Check sheet for the modelled part. Datum: model origin and axes. Units: mm. A direction names the side the tool comes from. Give positions to 0.01 mm unless a question says otherwise; leave off trailing zeros. Order: outer loops, then holes, each group sorted by start corner. A loop starts at its lowest first (then second) coordinate and runs counter-clockwise, first axis right, second up.
```python
from build123d import *

# Parameters (mm, degrees)
SKETCH1_W               = 190
SKETCH1_H               = 50
BOSS_EXTRUDE1_DEPTH     = 120
SHELL1_T                = 5
SKETCH3_R               = 6.75
CUT_EXTRUDE2_DEPTH      = 242.091269025
CUT_EXTRUDE2_DEPTH_BACK = 242.091269025
M3_CLEARANCE_HOLE1_D    = 3.4
SKETCH8_R               = 7.5
CUT_EXTRUDE4_DEPTH      = 168.705098312
CUT_EXTRUDE4_DEPTH_BACK = 168.705098312
SKETCH10_W              = 13.4
SKETCH10_H              = 7.3
CUT_EXTRUDE6_DEPTH      = 5
FILLET1_R               = 3
SKETCH11_W              = 98.43460289
SKETCH11_H              = 30
REVOLVE1_ANGLE          = 15
CUT_EXTRUDE7_REACH      = 271.031
SKETCH12_R              = 2.2
M3_CLEARANCE_HOLE3_D    = 3.4


with BuildPart() as part:
    # Sketch1 → Boss-Extrude1 (new, symmetric)
    with BuildSketch(Plane.XY):
        with Locations((0, 25)):
            Rectangle(SKETCH1_W, SKETCH1_H)
    extrude(amount=BOSS_EXTRUDE1_DEPTH, both=True)

    # Shell1
    shell1_openings = [part.faces().sort_by_distance(p)[0] for p in [
        (0, 50, 0),
    ]]
    offset(amount=SHELL1_T, openings=shell1_openings, kind=Kind.INTERSECTION)

    # Sketch3 → Cut-Extrude2 (cut, two sides)
    with BuildSketch(Plane(origin=(100, 0, 0), x_dir=(0, 0, -1), z_dir=(1, 0, 0))) as cut_extrude2_sk:
        with Locations(Location((0, 20, 0), (0, 0, 270))):
            Circle(SKETCH3_R)
    extrude(amount=CUT_EXTRUDE2_DEPTH, mode=Mode.SUBTRACT)
    extrude(cut_extrude2_sk.sketch, amount=-CUT_EXTRUDE2_DEPTH_BACK, mode=Mode.SUBTRACT)

    # M3 Clearance Hole1 (through all)
    with Locations(Plane.XY.offset(125)):
        with Locations((-80.25, 42), (79.75, 42)):
            Hole(M3_CLEARANCE_HOLE1_D / 2)

    # Sketch8 → Cut-Extrude4 (cut, two sides)
    with BuildSketch(Plane(origin=(0, 0, 0), x_dir=(0, 0, -1), z_dir=(1, 0, 0))) as cut_extrude4_sk:
        with Locations((30, 25)):
            Circle(SKETCH8_R)
    extrude(amount=CUT_EXTRUDE4_DEPTH, mode=Mode.SUBTRACT)
    extrude(cut_extrude4_sk.sketch, amount=-CUT_EXTRUDE4_DEPTH_BACK, mode=Mode.SUBTRACT)

    # Sketch10 → Cut-Extrude6 (cut)
    with BuildSketch(Plane(origin=(0, 0, -125), x_dir=(-1, 0, 0), z_dir=(0, 0, -1))):
        with Locations((-15.8, 3.65)):
            Rectangle(SKETCH10_W, SKETCH10_H)
    extrude(amount=-CUT_EXTRUDE6_DEPTH, mode=Mode.SUBTRACT)

    # Fillet1
    fillet1_edges = [part.edges().sort_by_distance(p)[0] for p in [
        (22.5, 0, -122.5),
        (22.5, 7.3, -122.5),
        (9.1, 7.3, -122.5),
        (9.1, 0, -122.5),
    ]]
    fillet(fillet1_edges, radius=FILLET1_R)

    # Sketch11 → Revolve1 (revolve)
    with BuildSketch(Plane(origin=(0, 0, -125), x_dir=(-1, 0, 0), z_dir=(0, 0, -1))):
        with Locations((0, 35)):
            Rectangle(SKETCH11_W, SKETCH11_H)
    revolve(axis=Axis((49.217301445, 20, -125), (-1, 0, 0)), revolution_arc=REVOLVE1_ANGLE)

    # Cut-Extrude7: up to this plane
    cut_extrude7_end = Plane(origin=(0, 0, -120), z_dir=(0, 0, -1))
    # Sketch12 → Cut-Extrude7 (cut, up to the surface)
    with BuildSketch(Plane(origin=(0, -29.910254038, -111.626587737), x_dir=(-1, 0, 0), z_dir=(0, -0.25881904510252135, -0.9659258262890682)), mode=Mode.PRIVATE) as cut_extrude7_sk1:
        with Locations(Location((-37.5, 71.670897164, 0), (0, 0, 90))):
            Circle(SKETCH12_R)
    cut_extrude7_tool1 = split(extrude(cut_extrude7_sk1.sketch, amount=-CUT_EXTRUDE7_REACH, mode=Mode.PRIVATE), bisect_by=cut_extrude7_end, keep=Keep.BOTH, mode=Mode.PRIVATE)
    cut_extrude7 = cut_extrude7_tool1.solids().sort_by_distance((37.5, 39.318517, -130.176381))[0]
    add(cut_extrude7, mode=Mode.SUBTRACT)

    # Mirror2: Cut-Extrude7 across plane
    add(cut_extrude7.mirror(Plane(origin=(0, 0, 0), x_dir=(0, 0, 1), z_dir=(1, 0, 0))), mode=Mode.SUBTRACT)

    # M3 Clearance Hole3 (through all)
    with Locations(Plane(origin=(0, 5, 0), x_dir=(1, 0, 0), z_dir=(0, 1, 0))):
        with Locations((-47.903181707, 25), (-86.25, 25), (-47.903181707, -25), (-86.25, -25), (25, -49.28), (47.903181707, -25), (86.25, -25), (86.25, 25), (47.903181707, 25), (25, 31.75), (-25, 31.75), (-25, -49.28)):
            Hole(M3_CLEARANCE_HOLE3_D / 2)


solid = part.part
```
Q1. Go/stop test with flat-tipped pins: P1, Ø2, axis at x = -25, z = -31.75, coming from the -Y side; P2, Ø3, axis at x = 30, y = 10.5, coming from the -Z side; P3, Ø4, axis at x = -47.9, z = 25, coming from the +Y side; P4, Ø4, axis at y = 34.5, z = -129, coming from the +X side. Record where each tip stops, or that it passes through.
Q2. Sectioned sample at A-A, the plane z = 32.5. Record the cut outline in (x, y), plus the area to 3 significant figures.
Q3. Tool access check on faces 1 (the flat face through (-1, 17, -125)), 2 (the flat face through (16, 7.3, -123)), 3 (the flat face through (-1, 25, 120)), 4 (the flat face through (-49.217, 39, -128)). Record the directions out of +Z, -Z, +X, -X, +Y, -Y that give a thin tool (end or side, any length) a straight path to the whole face; none if there is none.
Q4. Draft check along X on faces 5 (the flat face through (49.217, 39, -128)), 6 (the flat face through (-1, -5, 2)), 7 (the flat face through (-1, 0, -1)). Enter one of: pulls with the +X half, pulls with the -X half, needs draft (parallel to the pull), parting line crosses it, or undercut.
Q5. Sectioned sample at B-B, the plane x = 5.5. Record the cut outline in (y, z), plus the area to 3 significant figures.
Q6. Material ranges on line 1 (X direction, y = -2.75, z = -25); line 2 (Z direction, x = 25, y = -1.9); line 3 (Z direction, x = 86.25, y = -2.35), recorded low to high.
Filled in:
1. P1: passes through
1. P2: stops at z = -125
1. P3: stops at y = 0
1. P4: stops at x = 49.22
2. outline: (-100, -5) - (100, -5) - (100, 50) - (95, 50) - (95, 0) - (-95, 0) - (-95, 50) - (-100, 50) - close
2. area: 1,500 mm2
3. face 1: -Z, -Y
3. face 2: -Z
3. face 3: +Y
3. face 4: -Z, -X, +Y, -Y
4. face 5: pulls with the +X half
4. face 6: needs draft
4. face 7: undercut
5. outline: (-5, -125) - (20, -125) - (48.98, -132.76) arc R30 ccw to (50, -125) - (50, -120) - (0, -120) - (0, 120) - (50, 120) - (50, 125) - (-5, 125) - close
5. area: 1,870 mm2
6. line 1: x = -100 to -87.95, -84.55 to -49.6, -46.2 to 46.2, 49.6 to 84.55, 87.95 to 100
6. line 2: z = -125 to -33.45, -30.05 to 47.58, 50.98 to 125
6. line 3: z = -125 to -26.7, -23.3 to 23.3, 26.7 to 125
